```python
from build123d import *

# Parameters (mm, degrees)
F0_R     = 5
F1_DEPTH = 75
F2_R     = 3.45
F3_DEPTH = 20
F4_R     = 2.1
F5_DEPTH = 5
F6_R     = 2.1
F7_DEPTH = 10


with BuildPart() as f1:
    # F0 (on Top) → F1 (new body)
    with BuildSketch(Plane.XY):
        Circle(F0_R)
    extrude(amount=F1_DEPTH)

    # F2 (on face) → F3 (join)
    with BuildSketch(Plane.XY.offset(75)):
        Circle(F2_R)
    extrude(amount=F3_DEPTH)

    # F4 (on face) → F5 (join)
    with BuildSketch(Plane.XY.offset(95)):
        Circle(F4_R)
    extrude(amount=F5_DEPTH)

    # F6 (on face) → F7 (cut)
    with BuildSketch(Plane(origin=(0, 0, 0), x_dir=(1, 0, 0), z_dir=(0, 0, -1))):
        Circle(F6_R)
    extrude(amount=-F7_DEPTH, mode=Mode.SUBTRACT)


solid = f1.part
```
The listing builds one solid part. Answer for the finished solid, in the listing's coordinates (mm). A direction names the side the tool comes from. Give positions to 0.01 mm unless a question says otherwise; leave off trailing zeros. Order: outer loops, then holes, each group sorted by start corner. A loop starts at its lowest first (then second) coordinate and runs counter-clockwise, first axis right, second up. Notation, with made-up numbers: (85, 8) - (97, 8) arc R25 cw to (97, 46) - close; hole circle Ø3 at (76, -3.75). An arc over 180 degrees is marked (long way). Answer in a Markdown table with one row per item. Add a question column.
Q1. Which of the six approach directions +Z, -Z, +X, -X, +Y, -Y give full straight-line access (tool end or side, diameter ignored) to faces 4 (the flat face through (0, 0, 10)), 5 (the flat face through (1, -2.2, 0)), 6 (the flat face through (0, -2.3, 95))?
Q2. Find the intervals of material crossed by line 1 along Y through (x, z) = (0, 4.75); line 2 along Z through (x, y) = (0.75, -2.5); line 3 along X through (y, z) = (-0.25, 85.5), in increasing order. Write a range as [from, to].
Q3. Given P1, Ø6, axis at x = -1.5, z = 17.5, coming from the -Y side; P2, Ø3, axis at x = 2.5, z = 37.5, coming from the -Y side; P3, Ø3, axis at y = 2.5, z = 48, coming from the -X side; P4, Ø1, axis at x = -2, z = 50.5, coming from the +Y side, each flat-ended and moving along its own axis, determine where each tip first touches the part or whether it passes through.
Q4. For a pull along X with two mould halves and no side action, classify faces 1 (the cylindrical face through (2.003, -0.631, 4.93)), 2 (the cylindrical face through (-1.08, -4.88, 36.98)), 3 (the flat face through (0, 0, 100)) as released by +X, released by -X, zero draft, split by the parting line, or undercut.
Q5. The part is cut by section C-C (z = 15). Determine the outline of the cut face in (x, y), then the cut area to 3 significant figures.
Q6. The part is cut by section B-B (y = -1.25). Determine the outline of the cut face in (x, z), then the cut area to 3 significant figures.
Q7. The part is cut by section A-A (x = 0). Determine the outline of the cut face in (y, z), then the cut area to 3 significant figures.
Determined:
| question | item | result |
|---|---|---|
| 1 | face 4 | -Z |
| 1 | face 5 | -Z, +X, -X, +Y, -Y |
| 1 | face 6 | +Z |
| 2 | line 1 | y = [-5, -2.1], [2.1, 5] |
| 2 | line 2 | z = [0, 95] |
| 2 | line 3 | x = [-3.44, 3.44] |
| 3 | P1 | stops at y = -5 |
| 3 | P2 | stops at y = -4.9 |
| 3 | P3 | stops at x = -4.9 |
| 3 | P4 | stops at y = 4.77 |
| 4 | face 1 | undercut |
| 4 | face 2 | split by the parting line |
| 4 | face 3 | zero draft |
| 5 | outline | circle Ø10 at (0, 0) |
| 5 | area | 78.5 mm² |
| 6 | outline | (-4.84, 0) - (-1.69, 0) - (-1.69, 10) - (1.69, 10) - (1.69, 0) - (4.84, 0) - (4.84, 75) - (3.22, 75) - (3.22, 95) - (1.69, 95) - (1.69, 100) - (-1.69, 100) - (-1.69, 95) - (-3.22, 95) - (-3.22, 75) - (-4.84, 75) - close |
| 6 | area | 838 mm² |
| 7 | outline | (-5, 0) - (-2.1, 0) - (-2.1, 10) - (2.1, 10) - (2.1, 0) - (5, 0) - (5, 75) - (3.45, 75) - (3.45, 95) - (2.1, 95) - (2.1, 100) - (-2.1, 100) - (-2.1, 95) - (-3.45, 95) - (-3.45, 75) - (-5, 75) - close |
| 7 | area | 867 mm² |
